from build123d import *

# Parameters (mm, degrees)
SKETCH1_W               = 50
SKETCH1_H               = 50
BOSS_EXTRUDE1_DEPTH     = 1
SKETCH2_W               = 30
SKETCH2_H               = 15
BOSS_EXTRUDE2_DEPTH     = 15
SKETCH3_W               = 4
SKETCH3_H               = 8
CUT_EXTRUDE1_DEPTH      = 15
LPATTERN1_COUNT         = 5
LPATTERN1_PITCH         = 6
SKETCH4_W               = 28.997930891
SKETCH4_H               = 2
SKETCH4_H_2             = 2.5
SKETCH4_H_3             = 1
CUT_EXTRUDE2_DEPTH      = 2
CUT_EXTRUDE3_START      = -7
SKETCH4_3_W             = 28.997930891
SKETCH4_3_H             = 2
SKETCH4_3_H_2           = 2.5
CUT_EXTRUDE3_DEPTH      = 5
CUT_EXTRUDE4_START      = -15
SKETCH4_4_W             = 28.997930891
SKETCH4_4_H             = 2
CUT_EXTRUDE4_DEPTH      = 8
CUT_EXTRUDE5_DEPTH      = 1
SKETCH6_R               = 1.5
SKETCH6_W               = 2.5
SKETCH6_H               = 0.3
SKETCH6_W_2             = 0.3
SKETCH6_H_2             = 2.5
SKETCH6_H_3             = 1.1
SKETCH6_W_3             = 1.1
BOSS_EXTRUDE3_DEPTH     = 0.1
SKETCH6_3_R             = 1.5
BOSS_EXTRUDE4_DEPTH     = 1
SKETCH7_R               = 1.5
CUT_EXTRUDE6_DEPTH      = 73.284161474
SKETCH8_W               = 4
SKETCH8_H               = 1.5
BOSS_EXTRUDE5_DEPTH     = 1
LPATTERN2_COUNT         = 4
LPATTERN2_PITCH         = 3
MIRROR1_COPY_1_SKETCH_W = 4
MIRROR1_COPY_1_SKETCH_H = 1.5
MIRROR1_COPY_1_DEPTH    = 1
MIRROR1_COPY_2_SKETCH_W = 4
MIRROR1_COPY_2_SKETCH_H = 1.5
MIRROR1_COPY_2_DEPTH    = 1
MIRROR1_COPY_3_SKETCH_W = 4
MIRROR1_COPY_3_SKETCH_H = 1.5
MIRROR1_COPY_3_DEPTH    = 1
SKETCH9_W               = 5
SKETCH9_H               = 10
BOSS_EXTRUDE6_DEPTH     = 10
CUT_EXTRUDE7_DEPTH      = 10
SKETCH11_W              = 15
SKETCH11_H              = 5
BOSS_EXTRUDE7_DEPTH     = 10
CUT_EXTRUDE8_REACH      = 60.146
SKETCH13_W              = 2
SKETCH13_H              = 2
SKETCH13_R              = 0.995
BOSS_EXTRUDE9_DEPTH     = 7
LPATTERN3_COUNT         = 6
LPATTERN3_PITCH         = 2


with BuildPart() as part:
    # Sketch1 → Boss-Extrude1 (new body)
    with BuildSketch(Plane.XY):
        with Locations((25, 25)):
            Rectangle(SKETCH1_W, SKETCH1_H)
    extrude(amount=BOSS_EXTRUDE1_DEPTH)

    # Sketch2 → Boss-Extrude2 (add)
    with BuildSketch(Plane.XY.offset(1)):
        with Locations((25, 42.5)):
            Rectangle(SKETCH2_W, SKETCH2_H)
    extrude(amount=BOSS_EXTRUDE2_DEPTH)

    # Sketch3 → Cut-Extrude1 (cut)
    with BuildSketch(Plane.XY.offset(16)):
        with Locations((12.8, 46)):
            Rectangle(SKETCH3_W, SKETCH3_H)
    cut_extrude1 = extrude(amount=-CUT_EXTRUDE1_DEPTH, mode=Mode.SUBTRACT)

    # LPattern1: Cut-Extrude1 ×5
    with Locations(*[(i * LPATTERN1_PITCH, 0, 0) for i in range(1, LPATTERN1_COUNT)]):
        add(cut_extrude1, mode=Mode.SUBTRACT)

    # Sketch4 → Cut-Extrude2 (cut)
    with BuildSketch(Plane.XY.offset(16)):
        with Locations((25.001034555, 36)):
            Rectangle(SKETCH4_W, SKETCH4_H)
        with Locations((25.001034555, 38.25)):
            Rectangle(SKETCH4_W, SKETCH4_H_2)
        with Locations((25.001034555, 40)):
            Rectangle(SKETCH4_W, SKETCH4_H_3)
    extrude(amount=-CUT_EXTRUDE2_DEPTH, mode=Mode.SUBTRACT)

    # Sketch4<3> → Cut-Extrude3 (cut)
    with BuildSketch(Plane.XY.offset(16).offset(CUT_EXTRUDE3_START)):
        with Locations((25.001034555, 36)):
            Rectangle(SKETCH4_3_W, SKETCH4_3_H)
        with Locations((25.001034555, 38.25)):
            Rectangle(SKETCH4_3_W, SKETCH4_3_H_2)
    extrude(amount=CUT_EXTRUDE3_DEPTH, mode=Mode.SUBTRACT)

    # Sketch4<4> → Cut-Extrude4 (cut)
    with BuildSketch(Plane.XY.offset(16).offset(CUT_EXTRUDE4_START)):
        with Locations((25.001034555, 36)):
            Rectangle(SKETCH4_4_W, SKETCH4_4_H)
    extrude(amount=CUT_EXTRUDE4_DEPTH, mode=Mode.SUBTRACT)

    # Sketch5 → Cut-Extrude5 (cut)
    with BuildSketch(Plane.XZ.offset(-39.5)):
        Polygon((12.002069109, 14), (10.502069109, 14), (10.502069109, 12.5), align=None)
        Polygon((38, 14), (39.5, 14), (39.5, 12.5), align=None)
    extrude(amount=-CUT_EXTRUDE5_DEPTH, mode=Mode.SUBTRACT)

    # Sketch6 → Boss-Extrude3 (add)
    # profile 1 of 6: a face of its own
    with BuildSketch(Plane.XZ.offset(-39.5)):
        with Locations(Location((25.001034554, 11.5, 0), (0, 0, 270))):
            Circle(SKETCH6_R)
        with Locations((25.001034554, 11.5)):
            Rectangle(SKETCH6_W, SKETCH6_H, mode=Mode.SUBTRACT)
        with Locations((25.001034554, 11.5)):
            Rectangle(SKETCH6_W_2, SKETCH6_H_2, mode=Mode.SUBTRACT)
    # profile 2 of 6: a face of its own
    with BuildSketch(Plane.XZ.offset(-39.5)):
        with Locations((25.001034554, 10.8)):
            Rectangle(SKETCH6_W_2, SKETCH6_H_3)
    # profile 3 of 6: a face of its own
    with BuildSketch(Plane.XZ.offset(-39.5)):
        with Locations((25.701034554, 11.5)):
            Rectangle(SKETCH6_W_3, SKETCH6_H)
    # profile 4 of 6: a face of its own
    with BuildSketch(Plane.XZ.offset(-39.5)):
        with Locations((25.001034554, 12.2)):
            Rectangle(SKETCH6_W_2, SKETCH6_H_3)
    # profile 5 of 6: a face of its own
    with BuildSketch(Plane.XZ.offset(-39.5)):
        with Locations((25.001034554, 11.5)):
            Rectangle(SKETCH6_W_2, SKETCH6_H)
    # profile 6 of 6: a face of its own
    with BuildSketch(Plane.XZ.offset(-39.5)):
        with Locations((24.301034554, 11.5)):
            Rectangle(SKETCH6_W_3, SKETCH6_H)
    extrude(amount=BOSS_EXTRUDE3_DEPTH)

    # Sketch6<3> → Boss-Extrude4 (add)
    with BuildSketch(Plane.XZ.offset(-39.5)):
        with Locations(Location((25.001034554, 11.5, 0), (0, 0, 270))):
            Circle(SKETCH6_3_R)
        Polygon((25.151034554, 10.25), (24.851034554, 10.25), (24.851034554, 11.35), (23.751034554, 11.35), (23.751034554, 11.65), (24.851034554, 11.65), (24.851034554, 12.75), (25.151034554, 12.75), (25.151034554, 11.65), (26.251034554, 11.65), (26.251034554, 11.35), (25.151034554, 11.35), align=None, mode=Mode.SUBTRACT)
    extrude(amount=BOSS_EXTRUDE4_DEPTH)

    # Sketch7 → Cut-Extrude6 (cut, through all)
    with BuildSketch(Plane.XY.offset(1)):
        with Locations((48, 47)):
            Circle(SKETCH7_R)
        with Locations((48, 3)):
            Circle(SKETCH7_R)
        with Locations((2, 3)):
            Circle(SKETCH7_R)
        with Locations((2, 47)):
            Circle(SKETCH7_R)
    extrude(amount=-CUT_EXTRUDE6_DEPTH, mode=Mode.SUBTRACT)

    # Sketch8 → Boss-Extrude5 (add)
    with BuildSketch(Plane.XY.offset(1)):
        with Locations((47, 40.25)):
            Rectangle(SKETCH8_W, SKETCH8_H)
    boss_extrude5 = extrude(amount=BOSS_EXTRUDE5_DEPTH)

    # LPattern2: Boss-Extrude5 ×4
    with Locations(*[(0, -i * LPATTERN2_PITCH, 0) for i in range(1, LPATTERN2_COUNT)]):
        add(boss_extrude5)

    # Mirror1: Boss-Extrude5 across plane
    add(boss_extrude5.mirror(Plane(origin=(25, 0, 0), x_dir=(0, 0, 1), z_dir=(1, 0, 0))))

    # Mirror1 copy 1 sketch → Mirror1 copy 1 (add)
    with BuildSketch(Plane(origin=(50, -3, 1), x_dir=(-1, 0, 0), z_dir=(0, 0, 1))):
        with Locations((47, -40.25)):
            Rectangle(MIRROR1_COPY_1_SKETCH_W, MIRROR1_COPY_1_SKETCH_H)
    extrude(amount=MIRROR1_COPY_1_DEPTH)

    # Mirror1 copy 2 sketch → Mirror1 copy 2 (add)
    with BuildSketch(Plane(origin=(50, -6, 1), x_dir=(-1, 0, 0), z_dir=(0, 0, 1))):
        with Locations((47, -40.25)):
            Rectangle(MIRROR1_COPY_2_SKETCH_W, MIRROR1_COPY_2_SKETCH_H)
    extrude(amount=MIRROR1_COPY_2_DEPTH)

    # Mirror1 copy 3 sketch → Mirror1 copy 3 (add)
    with BuildSketch(Plane(origin=(50, -9, 1), x_dir=(-1, 0, 0), z_dir=(0, 0, 1))):
        with Locations((47, -40.25)):
            Rectangle(MIRROR1_COPY_3_SKETCH_W, MIRROR1_COPY_3_SKETCH_H)
    extrude(amount=MIRROR1_COPY_3_DEPTH)

    # Sketch9 → Boss-Extrude6 (add)
    with BuildSketch(Plane.XY.offset(1)):
        with Locations((46.5, 16)):
            Rectangle(SKETCH9_W, SKETCH9_H)
    boss_extrude6 = extrude(amount=BOSS_EXTRUDE6_DEPTH)

    # Sketch10 → Cut-Extrude7 (cut)
    with BuildSketch(Plane(origin=(0, 21, 0), x_dir=(1, 0, 0), z_dir=(0, 1, 0))):
        Polygon((45.2, -11), (44, -11), (44, -9), align=None)
    cut_extrude7 = extrude(amount=-CUT_EXTRUDE7_DEPTH, mode=Mode.SUBTRACT)

    # Mirror2: Boss-Extrude6, Cut-Extrude7 across plane
    add(boss_extrude6.mirror(Plane(origin=(25, 0, 0), x_dir=(0, 0, 1), z_dir=(1, 0, 0))))
    add(cut_extrude7.mirror(Plane(origin=(25, 0, 0), x_dir=(0, 0, 1), z_dir=(1, 0, 0))), mode=Mode.SUBTRACT)

    # Sketch11 → Boss-Extrude7 (add)
    with BuildSketch(Plane.XY.offset(1)):
        with Locations((17.5, 3.5)):
            Rectangle(SKETCH11_W, SKETCH11_H)
    extrude(amount=BOSS_EXTRUDE7_DEPTH)

    # Sketch12 → Cut-Extrude8 (cut, up to next)
    with BuildSketch(Plane(origin=(25, 0, 0), x_dir=(0, 0, -1), z_dir=(1, 0, 0)), mode=Mode.PRIVATE) as cut_extrude8_sk1:
        Polygon((-11, 5), (-11, 6), (-9, 6), align=None)
    cut_extrude8_tool1 = extrude(cut_extrude8_sk1.sketch, amount=-CUT_EXTRUDE8_REACH, mode=Mode.PRIVATE) & part.part
    add(cut_extrude8_tool1.solids().sort_by_distance((25, 5.666667, 10.333333))[0], mode=Mode.SUBTRACT)

    # Sketch13 → Boss-Extrude9 (add)
    with BuildSketch(Plane.XY.offset(1)):
        with Locations((28, 3.5)):
            Rectangle(SKETCH13_W, SKETCH13_H)
        with Locations((28, 3.5)):
            Circle(SKETCH13_R, mode=Mode.SUBTRACT)
    boss_extrude9 = extrude(amount=BOSS_EXTRUDE9_DEPTH)

    # LPattern3: Boss-Extrude9 ×6
    with Locations(*[(i * LPATTERN3_PITCH, 0, 0) for i in range(1, LPATTERN3_COUNT)]):
        add(boss_extrude9)


solid = part.part
Model file for the job. Use its own axes, mm. A direction names the side the tool comes from. Round coordinates to 2 decimals unless told otherwise and drop trailing zeros. Order: outer loops, then holes, each group sorted by start corner. A loop starts at its lowest first (then second) coordinate and runs counter-clockwise, first axis right, second up.
(1) Band-saw the part on A-A (x = 48). Give the number of separate pieces and of enclosed holes in the cut face, then the cut area to 3 significant figures.
(2) Drill centre lines: line 1 (Y direction, x = 48, z = 0.5); line 2 (X direction, y = 18.5, z = 2.5); line 3 (Y direction, x = 15.5, z = 6). Where is each one in solid material? Low to high.
(3) 3-axis set-ups, long thin cutter, end or side, ignore diameter. For faces 1 (the face through (17.6, 5.5, 10)), 2 (the face through (38, 4, 1)), 3 (the face through (10, 3, 6)): which of +Z, -Z, +X, -X, +Y, -Y reach the whole face in a straight line?
(4) Pull direction X, two halves, no side cores. Call faces 4 (the face through (31, 42, 9)), 5 (the face through (10.502, 37, 10)), 6 (the face through (49, 16, 6)), 7 (the face through (17, 6, 5)): released by +X, released by -X, zero draft, split by the parting line, or undercut.
(5) Band-saw the part on D-D (x = 30). List the corners of the cut face in (y, z) (3 decimals).
(6) Band-saw the part on B-B (y = 16). List the corners of the cut face in (x, z).
(7) Pin check, flat tips, straight feed: pin 1 (0.8 mm diameter, centred on y = 37.5, z = 1.5, fed in from -X); pin 2 (0.8 mm diameter, centred on x = 47, y = 37, fed in from +Z); pin 3 (4 mm diameter, centred on y = 47, z = 10, fed in from +X); pin 4 (4 mm diameter, centred on y = 8, z = 12, fed in from -X). Stop position of each tip, or through.
Verdict:
1. separate pieces: 3
1. enclosed holes: 0
1. area: 150 mm2
2. line 1: y = 0 to 1.5, 4.5 to 45.5, 48.5 to 50
2. line 2: x = 1 to 6, 44 to 49
2. line 3: y = 1 to 6, 37 to 50
3. face 1: +Z, +X, -X
3. face 2: +Z
3. face 3: +Z, -X, +Y, -Y
4. face 4: undercut
4. face 5: undercut
4. face 6: released by +X
4. face 7: zero draft
5. outline: (0, 0) - (50, 0) - (50, 1) - (42, 1) - (42, 16) - (40.5, 16) - (40.5, 14) - (39.5, 14) - (39.5, 9) - (37, 9) - (37, 1) - (4.5, 1) - (4.5, 8) - (4.495, 8) - (4.495, 1) - (2.505, 1) - (2.505, 8) - (2.5, 8) - (2.5, 1) - (0, 1) - close
6. outline: (0, 0) - (50, 0) - (50, 1) - (49, 1) - (49, 11) - (45.2, 11) - (44, 9) - (44, 1) - (6, 1) - (6, 9) - (4.8, 11) - (1, 11) - (1, 1) - (0, 1) - close
7. pin 1: stops at x = 1
7. pin 2: stops at z = 2
7. pin 3: stops at x = 40
7. pin 4: passes through
